CAD build for the part. Positions are in the model's coordinates, mm. Face numbers are marked on the shaded views. A direction names the side the tool comes from. Give positions to 0.01 mm unless a question says otherwise; leave off trailing zeros. Write each loop counter-clockwise with the first axis right and the second up, starting at its lowest first coordinate (ties: lowest second). Pieces come first, ordered by that corner, then holes. Notation, with made-up numbers: (-9, 3.5) - (5, 3.5) arc R15 ccw to (5, 18.5) - close; hole circle Ø8 at (-32, 50). An arc over 180 degrees is marked (long way). Answer as a JSON object with one key per item and string values.
Autodesk Inventor part; units mm, degrees
ref_plane "YZ Plane" through (0, 0, 0) normal (1, 0, 0) x (0, 1, 0)
ref_plane "XZ Plane" through (0, 0, 0) normal (0, 1, 0) x (-1, 0, 0)
ref_plane "XY Plane" through (0, 0, 0) normal (0, 0, 1) x (1, 0, 0)
sketch "Эскиз3" plane through (0, 0, 0) normal (0, 0, 1) x (1, 0, 0)
  circle A0 centre (0, 0) radius 41.5
  line L0 (12.5, -11.0597) -> (-12.5, -11.0597)
  line L1 (-12.5, -11.0597) -> (-12.5, -28.0597)
  line L2 (-12.5, -11.0597) -> (12.5, -11.0597)
  line L3 (12.5, -11.0597) -> (12.5, -28.0597)
  line L4 (12.5, -28.0597) -> (-12.5, -28.0597)
  line L5 (-12.5, -28.0597) -> (-12.5, -11.0597)
  dimension "d9" = 83
  dimension "d10" = 25
  dimension "d11" = 17
  dimension "d13" = 25
  dimension "d14" = 17
  dimension "d15" = 12.5
extrude "Выдавливание3" add sketch "Эскиз3" along normal blind 3
sketch "Эскиз4" plane through (0, 0, 3) normal (0, 0, 1) x (1, 0, 0)
  arc A0 (5.7629, -8.6636) -> (-4.709, -8.7124) centre (0.4132, 15.7598) ccw
  circle A1 centre (0.4132, 15.7598) radius 1.5338
  point P0 (0, 0)
extrude "Выдавливание4" cut sketch "Эскиз4" against normal blind 3
sketch "Эскиз5" plane through (0, 0, 3) normal (0, 0, 1) x (1, 0, 0)
  line L0 (28.2027, -2.4247) -> (31.5626, 4.2424)
  circle A0 centre (31.5626, 0.0623) radius 2.5
  point P0 (0, 0)
  dimension "d20" = 5
extrude "Выдавливание5" cut sketch "Эскиз5" against normal blind 3
sketch "Эскиз6" plane through (0, 0, 3) normal (0, 0, 1) x (1, 0, 0)
  circle A0 centre (0.4132, 15.7598) radius 1.5338
  point P0 (0, 0)
extrude "Выдавливание6" add sketch "Эскиз6" against normal blind 3
sketch "Эскиз7" plane through (0, 0, 3) normal (0, 0, 1) x (1, 0, 0)
  circle A0 centre (10.5, -7.8097) radius 1.25
  circle A1 centre (-10.5, -7.8097) radius 1.25
  circle A2 centre (-10.5, -31.3097) radius 1.25
  circle A3 centre (10.5, -31.3097) radius 1.25
  point P0 (0, 0)
extrude "Выдавливание7" cut sketch "Эскиз7" against normal blind 3
sketch "Эскиз8" plane through (0, 0, 0) normal (0, 0, -1) x (-1, 0, 0)
  line L0 (-18.7254, 8.2596) -> (19.2746, 8.2596)
  line L1 (-18.7254, 8.2596) -> (19.2746, 8.2596)
  line L2 (19.2746, 8.2596) -> (19.2746, 5.2596)
  line L3 (19.2746, 5.2596) -> (-18.7254, 5.2596)
  line L4 (-18.7254, 5.2596) -> (-18.7254, 8.2596)
  point P0 (0, 0)
  dimension "d27" = 3
extrude "Выдавливание8" add sketch "Эскиз8" along normal blind 56
sketch "Эскиз9" plane through (-19.2746, 8.2596, 0) normal (0, 1, 0) x (1, 0, 0)
  circle A0 centre (29, 41.5) radius 1.6
  circle A1 centre (22.71, 4.4641) radius 1.6
  point P0 (19.2746, 0)
extrude "Выдавливание9" cut sketch "Эскиз9" against normal blind 56
sketch "Эскиз10" plane through (-19.2746, 5.2596, 0) normal (0, -1, 0) x (1, 0, 0)
  line L0 (0, 0) -> (38, 0)
  line L1 (38, 0) -> (38, -60) construction
  point P0 (19.2746, 0)
  dimension "d32" = 60
sketch "Эскиз11" plane through (0, 0, -56) normal (0, 0, -1) x (-1, 0, 0)
  circle A0 centre (0, 0) radius 41.5
  line L0 (-18.7254, 5.2596) -> (19.2746, 5.2596)
  line L1 (19.2746, 5.2596) -> (19.2746, 8.2596)
  line L2 (19.2746, 8.2596) -> (-18.7254, 8.2596)
  line L3 (-18.7254, 8.2596) -> (-18.7254, 5.2596)
  line L4 (-18.7254, 5.2596) -> (-18.7254, 8.2596)
  line L5 (-18.7254, 8.2596) -> (19.2746, 8.2596)
  line L6 (19.2746, 8.2596) -> (19.2746, 13.2596)
  line L7 (19.2746, 13.2596) -> (-18.7254, 13.2596)
  line L8 (-18.7254, 13.2596) -> (-18.7254, 8.2596)
  dimension "d33" = 5
extrude "Выдавливание10" add sketch "Эскиз11" against normal blind 3
sketch "Эскиз12" plane through (0, 0, 0) normal (0, 0, -1) x (-1, 0, 0)
  circle A0 centre (0, 0) radius 41.5
  line L0 (-6.5, -33.0597) -> (-6.5, -30.5597)
  line L1 (6.5, -33.0597) -> (6.5, -30.5597)
  line L2 (-6.5, -35.5314) -> (6.5, -35.5314)
  line L3 (6.5, -35.5314) -> (6.5, -37.9075)
  line L4 (6.5, -37.9075) -> (-6.5, -37.9075)
  line L5 (-6.5, -37.9075) -> (-6.5, -35.5314)
extrude "Выдавливание11" add sketch "Эскиз12" along normal blind 54.75 contours L2 L3 L4 L5
fillet "Сопряжение1" radius 5 8 edges at (-19.2746, 6.7596, 0) (18.7254, 6.7596, 0) (6.5, -36.7195, 0) (-6.5, -36.7195, 0) (-6.5, -36.7195, -53) (-19.2746, 6.7596, -53) (6.5, -36.7195, -53) (18.7254, 6.7596, -53)
equation "\"d13\" = d10"
equation "\"d14\" = d11"
properties part number "top2"
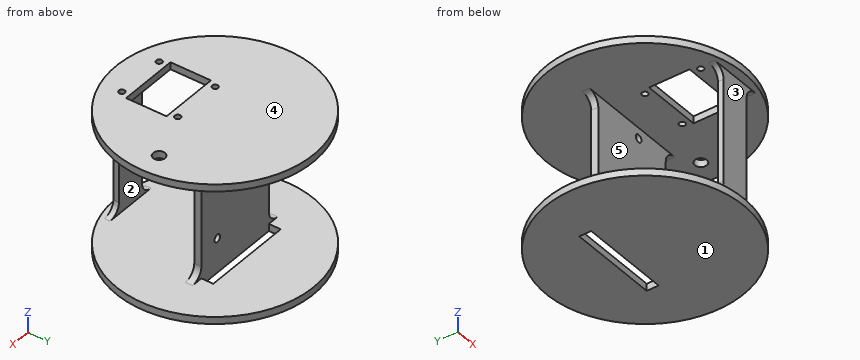
Item 1: Which spindle directions (+Z, -Z, +X, -X, +Y, -Y) get a long thin tool onto all of the face, cutting with end or side? Do the marked faces 4 and 5. Say none if no direction does.
Entries:
{"face 4": "+Z, +X, -X, +Y, -Y", "face 5": "+X, -X"}
Item 2: Cut at C-C (x = -23). Give the cut face in (y, z), and give its area (3 significant figures).
Entries:
{"outline": "(-34.54, -56) - (34.54, -56) - (34.54, -53) - (8.26, -53) - (8.26, -52.83) - (5.26, -52.83) - (5.26, -53) - (-34.54, -53) - close; (-34.54, 0) - (5.26, 0) - (5.26, -0.17) - (8.26, -0.17) - (8.26, 0) - (34.54, 0) - (34.54, 3) - (-34.54, 3) - close", "area": "416 mm2"}
Item 3: Mould opens along Y. For the marked faces 1, 2 and 3 say: +Y half, -Y half, draft (parallel to the pull), parting line (faces both ways), or undercut.
Entries:
{"face 1": "draft", "face 2": "undercut", "face 3": "-Y half"}
Item 4: Cut at D-D (y = -24). Give the cut face in (x, z), and give its area (3 significant figures).
Entries:
{"outline": "(-33.86, -56) - (33.86, -56) - (33.86, -53) - (-33.86, -53) - close; (-33.86, 0) - (-12.5, 0) - (-12.5, 3) - (-33.86, 3) - close; (12.5, 0) - (33.86, 0) - (33.86, 3) - (12.5, 3) - close", "area": "331 mm2"}
Item 5: Cut at B-B (z = -41.5). Give the cut face in (x, y).
Entries:
{"outline": "(-19.27, 5.26) - (8.13, 5.26) - (8.13, 8.26) - (-19.27, 8.26) - close; (-6.5, -37.91) - (6.5, -37.91) - (6.5, -35.53) - (-6.5, -35.53) - close; (11.33, 5.26) - (18.73, 5.26) - (18.73, 8.26) - (11.33, 8.26) - close"}
Item 6: Probe line 1 (Z direction, x = -20, y = -11.5); line 2 (Y direction, x = -10, z = 2); line 3 (Y direction, x = 10.5, z = 2.2). List the from-to ranges inside material, lowest first. Write a range as from..to.
Entries:
{"line 1": "-56..-53, 0..3", "line 2": "-40.28..-32.46, -30.16..-28.06, -11.06..-8.96, -6.66..40.28", "line 3": "-40.15..-32.56, -30.06..-28.06, -11.06..-9.06, -6.56..40.15"}
Item 7: Flat gauge pins, fed straight in: P1, Ø3.5, axis at x = 3.44, z = -4.46, coming from the +Y side; P2, Ø1.2, axis at y = -36.5, z = -19.5, coming from the +X side; P3, Ø1.5, axis at y = 6.5, z = -35.5, coming from the -X side; P4, Ø12, axis at x = -13, y = 9, coming from the -Z side. Where does each tip first touch, or does it go through?
Entries:
{"P1": "y = 8.26", "P2": "x = 6.5", "P3": "x = -19.27", "P4": "z = -56"}
Item 8: Cut at A-A (z = -23.5). Give the cut face in (x, y), and give its area (3 significant figures).
Entries:
{"outline": "(-19.27, 5.26) - (18.73, 5.26) - (18.73, 8.26) - (-19.27, 8.26) - close; (-6.5, -37.91) - (6.5, -37.91) - (6.5, -35.53) - (-6.5, -35.53) - close", "area": "145 mm2"}
